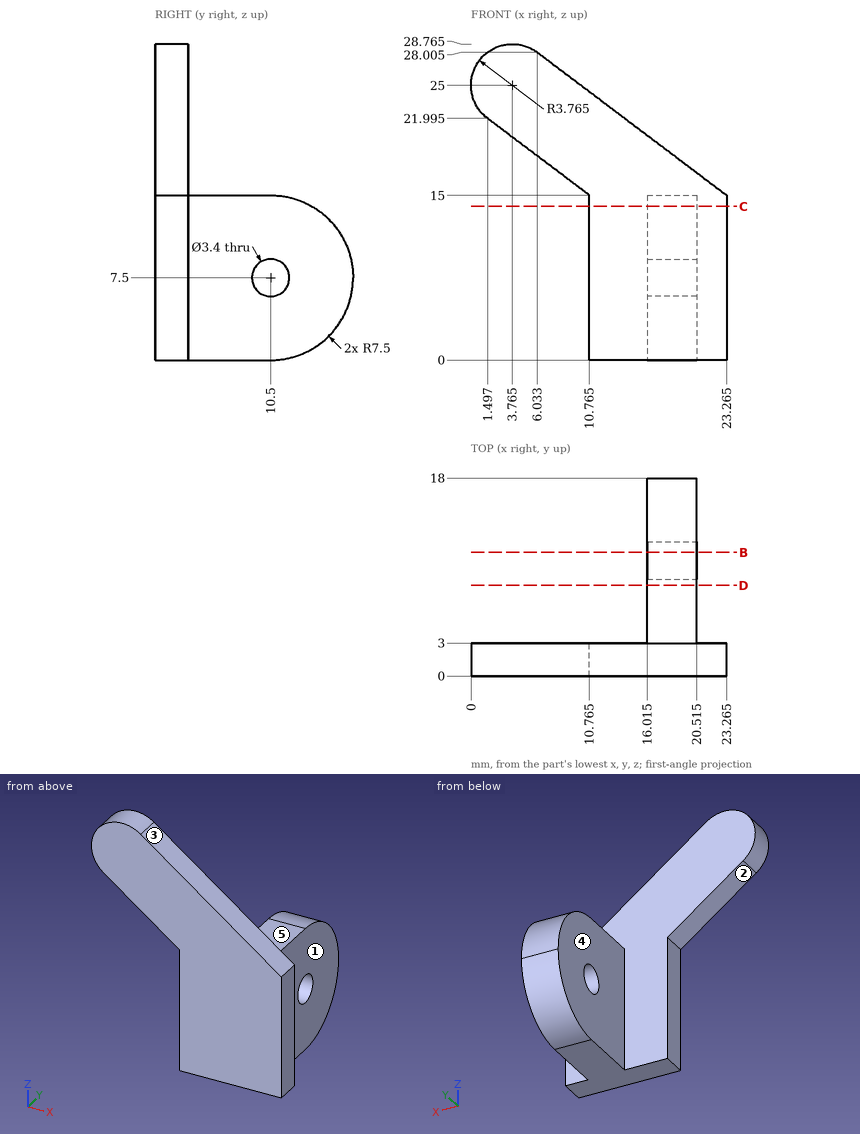
The figure shows three views and two pictorial views of one solid part (mm, origin at its lowest corner). Answer the questions. A direction names the side the tool comes from. Give positions to 0.01 mm unless a question says otherwise; leave off trailing zeros. Write each loop counter-clockwise with the first axis right and the second up, starting at its lowest first coordinate (ties: lowest second). Pieces come first, ordered by that corner, then holes. Notation, with made-up numbers: (3.25, 21) - (28.25, 21) arc R37 cw to (28.25, 60) - close; hole circle Ø7 at (64.25, 35). An arc over 180 degrees is marked (long way). Use one line per item in the form item = value. Start each with the question number.
1) Find section B-B on y = 11.25. Determine the outline of the cut face in (x, z) (1 decimal).
2) Flat-ended cylindrical pins translate along their axes: pin 1 Ø4.5 at (y, z) = (8, 11) entering from +X (3 decimals); pin 2 Ø8 at (x, z) = (4.5, 7.5) entering from +Y; pin 3 Ø6 at (x, z) = (8.5, 8.5) entering from +Y; pin 4 Ø10 at (y, z) = (4.5, 5.5) entering from +X (3 decimals). Find the tip coordinate at first contact, or state that the pin passes through.
3) Find section D-D on y = 8.25. Determine the outline of the cut face in (x, z) (3 decimals).
4) Find section C-C on z = 14. Determine the outline of the cut face in (x, y) (1 decimal).
5) A tool of negligible diameter and unlimited length cuts with its end or side. For the marked faces 1, 2, 3, 4 and 5, from which of +Z, -Z, +X, -X, +Y, -Y can it reach the whole face along a straight path? Write none if from no direction.
6) Consider line 1 along Y through (x, z) = (17.9, 7.5); line 2 along Y through (x, z) = (15, 14.25); line 3 along Z through (x, y) = (17, 12). Determine where each line is inside the solid, lowest interval first. Write a range as from..to.
Geometry results:
q1.outline = (16, 0) - (20.5, 0) - (20.5, 6) - (16, 6) - close; (16, 9) - (20.5, 9) - (20.5, 15) - (16, 15) - close
q2.pin_1 = 20.515
q2.pin_2 = through
q2.pin_3 = 3
q2.pin_4 = 23.265
q3.outline = (16.015, 0) - (20.515, 0) - (20.515, 15) - (16.015, 15) - close
q4.outline = (10.8, 0) - (23.3, 0) - (23.3, 3) - (20.5, 3) - (20.5, 14.2) - (16, 14.2) - (16, 3) - (10.8, 3) - close
q5.face_1 = +Z, -Z, +X, +Y
q5.face_2 = -Z, -X, +Y, -Y
q5.face_3 = +Z, +X, +Y, -Y
q5.face_4 = +Z, -Z, -X, +Y
q5.face_5 = +Z, +X, -X, +Y
q6.line_1 = 0..8.8, 12.2..18
q6.line_2 = 0..3
q6.line_3 = 0.15..6.7, 8.3..14.85
